from build123d import *
from build123d.topology import SkipClean

# Parameters (mm, degrees)
SKETCH4_W                = 20
SKETCH4_H                = 22
SKETCH4_R                = 4.75
BOSS_EXTRUDE2_DEPTH      = 30
CUT_EXTRUDE1_DEPTH       = 30
BOSS_EXTRUDE3_START      = 1
SKETCH11_W               = 20
SKETCH11_H               = 30
SKETCH11_R               = 4.2
BOSS_EXTRUDE3_DEPTH      = 1
SKETCH12_W               = 20
SKETCH12_H               = 30
SKETCH12_R               = 4.2
BOSS_EXTRUDE4_DEPTH      = 1
CUT_EXTRUDE2_DEPTH       = 10.75
SKETCH16_R               = 12.2
BOSS_EXTRUDE7_DEPTH      = 2
CUT_EXTRUDE3_START       = -2
SKETCH18_R               = 4.75
CUT_EXTRUDE3_DEPTH       = 2
BOSS_EXTRUDE8_START      = 3
SKETCH19_R               = 12.2
SKETCH19_R_2             = 10.4
SKETCH19_R_3             = 8.75
SKETCH19_R_4             = 4.75
BOSS_EXTRUDE8_DEPTH      = 3
SKETCH21_W               = 20
SKETCH21_H               = 24
SKETCH21_R               = 4.75
BOSS_EXTRUDE9_DEPTH      = 5
FILLET1_R                = 5
CUT_EXTRUDE12_DEPTH      = 44.205092
CUT_EXTRUDE12_DEPTH_BACK = 44.205092


with BuildPart() as part:
    # Sketch4 → Boss-Extrude2 (new body)
    with BuildSketch(Plane.XY):
        Rectangle(SKETCH4_W, SKETCH4_H)
        Circle(SKETCH4_R, mode=Mode.SUBTRACT)
    extrude(amount=-BOSS_EXTRUDE2_DEPTH)

    # Sketch7 → Cut-Extrude1 (cut)
    with BuildSketch(Plane.XZ.offset(11)):
        with BuildLine():
            ThreePointArc((4.2, -15), (2.969848, -12.030152), (0, -10.8))
            Line((0, -10.8), (0, -19.2))
            ThreePointArc((0, -19.2), (2.969848, -17.969848), (4.2, -15))
        make_face()
        with BuildLine():
            Line((0, -19.2), (0, -10.8))
            ThreePointArc((0, -10.8), (-4.2, -15), (0, -19.2))
        make_face()
    extrude(amount=-CUT_EXTRUDE1_DEPTH, mode=Mode.SUBTRACT)

    # Sketch11 → Boss-Extrude3 (add)
    with BuildSketch(Plane.XZ.offset(11).offset(BOSS_EXTRUDE3_START)):
        with Locations((0, -15)):
            Rectangle(SKETCH11_W, SKETCH11_H)
        with Locations((0, -15)):
            Circle(SKETCH11_R, mode=Mode.SUBTRACT)
    extrude(amount=-BOSS_EXTRUDE3_DEPTH)

    # Sketch12 → Boss-Extrude4 (add)
    with SkipClean():  # the faces are left unmerged after this step: merging them gives an invalid solid
        with BuildSketch(Plane(origin=(0, 11, 0), x_dir=(1, 0, 0), z_dir=(0, 1, 0))):
            with Locations((0, 15)):
                Rectangle(SKETCH12_W, SKETCH12_H)
            with Locations((0, 15)):
                Circle(SKETCH12_R, mode=Mode.SUBTRACT)
        extrude(amount=BOSS_EXTRUDE4_DEPTH)

    # Sketch9 → Cut-Extrude2 (cut, symmetric)
    with SkipClean():  # the faces are left unmerged after this step: merging them gives an invalid solid
        with BuildSketch(Plane(origin=(0, 0, 0), x_dir=(-1, 0, 0), z_dir=(0, -1, 0))):
            Polygon((7.216878, 15), (3.608439, 21.25), (-3.608439, 21.25), (-7.216878, 15), (-3.608439, 8.75), (3.608439, 8.75), align=None)
        extrude(amount=CUT_EXTRUDE2_DEPTH, both=True, mode=Mode.SUBTRACT)

    # Sketch16 → Boss-Extrude7 (add)
    with SkipClean():  # the faces are left unmerged after this step: merging them gives an invalid solid
        with BuildSketch(Plane.XY):
            with Locations(Location((0, 0, 0), (0, 0, 145.051986))):
                Circle(SKETCH16_R)
        extrude(amount=BOSS_EXTRUDE7_DEPTH)

    # Sketch18 → Cut-Extrude3 (cut)
    with SkipClean():  # the faces are left unmerged after this step: merging them gives an invalid solid
        with BuildSketch(Plane(origin=(0, 0, 0), x_dir=(-1, 0, 0), z_dir=(0, 0, -1)).offset(CUT_EXTRUDE3_START)):
            with Locations(Location((0, 0, 0), (0, 0, 139.435238))):
                Circle(SKETCH18_R)
        extrude(amount=CUT_EXTRUDE3_DEPTH, mode=Mode.SUBTRACT)

    # Sketch19 → Boss-Extrude8 (add)
    # profile 1 of 2: a face of its own
    with SkipClean():  # the faces are left unmerged after this step: merging them gives an invalid solid
        with BuildSketch(Plane.XY.offset(2).offset(BOSS_EXTRUDE8_START)):
            with Locations(Location((0, 0, 0), (0, 0, 145.051986))):
                Circle(SKETCH19_R)
            Circle(SKETCH19_R_2, mode=Mode.SUBTRACT)
        # profile 2 of 2: a face of its own
        with BuildSketch(Plane.XY.offset(2).offset(BOSS_EXTRUDE8_START)):
            Circle(SKETCH19_R_3)
            Circle(SKETCH19_R_4, mode=Mode.SUBTRACT)
        extrude(amount=-BOSS_EXTRUDE8_DEPTH)

    # Sketch21 → Boss-Extrude9 (add)
    with SkipClean():  # the faces are left unmerged after this step: merging them gives an invalid solid
        with BuildSketch(Plane(origin=(0, 0, -30), x_dir=(-1, 0, 0), z_dir=(0, 0, -1))):
            Rectangle(SKETCH21_W, SKETCH21_H)
            with Locations(Location((0, 0, 0), (0, 0, 180))):
                Circle(SKETCH21_R, mode=Mode.SUBTRACT)
        extrude(amount=BOSS_EXTRUDE9_DEPTH)

    # Fillet1
    fillet1_edges = [part.edges().sort_by_distance(p)[0] for p in [
        (10, 0, -35),
        (-10, 0, -35),
    ]]
    fillet(fillet1_edges, radius=FILLET1_R - 0.0001)  # a hair under: the kernel refuses the full size

    # Sketch27 → Cut-Extrude12 (cut, two sides: drawn at the far end of the back side and taken through both)
    with BuildSketch(Plane.ZY.offset(10).offset(-CUT_EXTRUDE12_DEPTH_BACK)):
        Polygon((-15, 10.75), (-8.8, 10.75), (-8.8, 4.75), (-21.2, 4.75), (-21.2, 10.75), align=None)
        Polygon((-21.2, -10.75), (-21.2, -4.75), (-8.8, -4.75), (-8.8, -10.75), (-15, -10.75), align=None)
    extrude(amount=CUT_EXTRUDE12_DEPTH + CUT_EXTRUDE12_DEPTH_BACK, mode=Mode.SUBTRACT)


solid = part.part
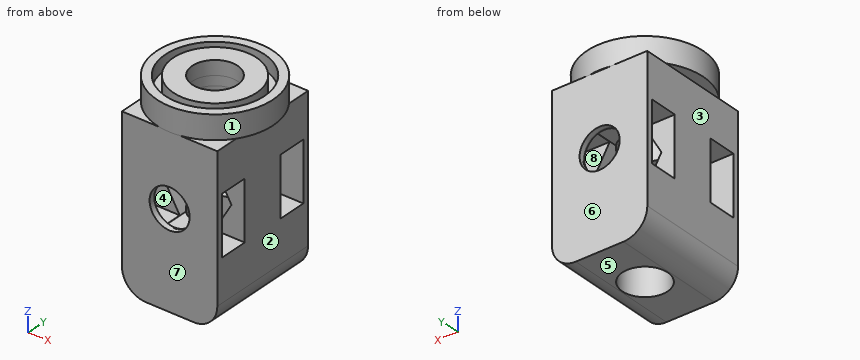
The listing builds one solid part. Answer for the finished solid, in the listing's coordinates (mm). Face numbers are marked on the shaded views. A direction names the side the tool comes from. Coordinates: 2 decimals unless noted, no trailing zeros. Loops run counter-clockwise (first coordinate to the right, second up) from the corner with the lowest first, then second, coordinate; pieces in that order, holes last. Notation, with made-up numbers: M 37.25,76.25 L 57.25,76.25 A13 cw 57.25,93.25 Z; hole C -23.75,-24.5 d2. An arc over 180 degrees is marked long. Answer in a Markdown table with one row per item.
1) Which of the six approach directions +Z, -Z, +X, -X, +Y, -Y give full straight-line access (tool end or side, diameter ignored) to the marked faces 1, 2, 3 and 4?
Answers below:
| item | result |
|---|---|
| face 1 | +Z |
| face 2 | -Z, +X, +Y, -Y |
| face 3 | -Z, -X, +Y, -Y |
| face 4 | +X, -X |
2) Find section B-B (z = -32). Determine the outline of the cut face in (x, y).
Answers below:
| item | result |
|---|---|
| outline | M -9.58,-12 L 9.58,-12 L 9.58,12 L -9.58,12 Z; hole C 0,0 d9.5 |
3) Determine the mould class of the marked faces 5, 6, 7 and 8 for opening direction Y: released by +Y, released by -Y, zero draft, split by the parting line, or undercut.
Answers below:
| item | result |
|---|---|
| face 5 | zero draft |
| face 6 | released by +Y |
| face 7 | released by -Y |
| face 8 | undercut |
4) Find the intervals of material crossed by probe 1 along Y at (x, z) = (-9.25, -10); probe 2 along Y at (x, z) = (0, 3.1); probe 3 along X at (y, z) = (0, -26.25), in increasing order.
Answers below:
| item | result |
|---|---|
| probe 1 | -12 to -10.75, -4.75 to 4.75, 10.75 to 12 |
| probe 2 | -12.2 to -10.4, -8.75 to -4.75, 4.75 to 8.75, 10.4 to 12.2 |
| probe 3 | -10 to -4.75, 4.75 to 10 |
5) Find section A-A (y = 0). Determine the outline of the cut face in (x, z).
Answers below:
| item | result |
|---|---|
| outline | M -12.2,0 L -10,0 L -10,-30 A5 ccw -5,-35 L -4.75,-35 L -4.75,-19.27 L -7.22,-15 L -4.75,-10.73 L -4.75,5 L -8.75,5 L -8.75,2 L -10.4,2 L -10.4,5 L -12.2,5 Z; M 4.75,-35 L 5,-35 A5 ccw 10,-30 L 10,0 L 12.2,0 L 12.2,5 L 10.4,5 L 10.4,2 L 8.75,2 L 8.75,5 L 4.75,5 L 4.75,-10.73 L 7.22,-15 L 4.75,-19.27 Z |
6) Given pin 1 (5 mm diameter, centred on x = -5.5, z = -7.5, fed in from +Y); pin 2 (1.9 mm diameter, centred on x = -7, z = -18, fed in from -Y); pin 3 (1.8 mm diameter, centred on x = 7.5, y = 9, fed in from -Z), each flat-ended and moving along its own axis, determine where each tip first touches the part or whether it passes through.
Answers below:
| item | result |
|---|---|
| pin 1 | y = 12 |
| pin 2 | y = -12 |
| pin 3 | z = -34.74 |
